```python
from build123d import *

# Parameters (mm, degrees)
BOSS_EXTRU_1_DEPTH = 10


with BuildPart() as part:
    # Esquisse1 → Boss.-Extru.1 (new body)
    with BuildSketch(Plane(origin=(0, 0, 0), x_dir=(1, 0, 0), z_dir=(0, 1, 0))):
        with BuildLine():
            Line((112.426746773, 8.058530984), (208.426746773, 8.058530984))
            Line((208.426746773, 8.058530984), (214.268189678, 17.812491045))
            ThreePointArc((214.268189678, 17.812491045), (206.831645665, 27.458673867), (208.340233589, 39.544830921))
            Line((208.340233589, 39.544830921), (290.262052013, 184.417099293))
            ThreePointArc((290.262052013, 184.417099293), (299.910234809, 191.958577714), (312.065160821, 190.468912764))
            Line((312.065160821, 190.468912764), (318.76181291, 202.523064381))
            Line((318.76181291, 202.523064381), (269.51839591, 284.931109389))
            Line((269.51839591, 284.931109389), (258.259283583, 284.517680144))
            Line((258.259283583, 284.517680144), (258.259283583, 282.707559459))
            ThreePointArc((258.259283583, 282.707559459), (253.572992082, 271.39385096), (242.259283583, 266.707559459))
            Line((242.259283583, 266.707559459), (75.828641942, 266.707559459))
            ThreePointArc((75.828641942, 266.707559459), (64.656934191, 271.253610536), (59.833620697, 282.308441218))
            Line((59.833620697, 282.308441218), (59.827222367, 282.56486004))
            Line((59.827222367, 282.56486004), (48.463462476, 282.281304065))
            Line((48.463462476, 282.281304065), (1.209576466, 198.716537226))
            Line((1.209576466, 198.716537226), (7.119810651, 189.400838648))
            ThreePointArc((7.119810651, 189.400838648), (19.083596298, 190.931024082), (28.716557185, 183.672945892))
            Line((28.716557185, 183.672945892), (114.087531018, 40.806031234))
            ThreePointArc((114.087531018, 40.806031234), (115.621763688, 27.817531222), (106.953563168, 18.023793314))
            Line((106.953563168, 18.023793314), (112.426746773, 8.058530984))
        make_face()
    extrude(amount=BOSS_EXTRU_1_DEPTH)


solid = part.part
```
Input: part model. Units: mm. Frame: model coordinates. A direction names the side the tool comes from. Round coordinates to 2 decimals unless told otherwise and drop trailing zeros. Write each loop counter-clockwise with the first axis right and the second up, starting at its lowest first coordinate (ties: lowest second). Pieces come first, ordered by that corner, then holes. Notation, with made-up numbers: M 33.5,53.5 L 85.5,53.5 A23 cw 85.5,65.5 Z; hole C 75,41 d2. An arc over 180 degrees is marked long. Write each question's results on one line, items separated by ' | '.
Q1. Draft query along X for faces 3 (the face through (160, 5, -266.708)), 4 (the face through (294.485, 4.93, -243.15)), 5 (the face through (158, 0, -148)). Return one class per face: released by +X, released by -X, zero draft, split by the parting line, or undercut.
Results:
face 3: undercut | face 4: released by +X | face 5: zero draft
Q2. Line query: line 1 along Z through (x, y) = (179, 1.25); line 2 along Z through (x, y) = (84, 3.5); line 3 along X through (y, z) = (9.75, -82.5). Output: solid intervals per line, ascending.
Results:
line 1: z = -266.71 to -8.06 | line 2: z = -266.71 to -91.16 | line 3: x = 89.17 to 232.63
Q3. Access query for faces 1 (the face through (263.968, 4.93, -284.727)), 2 (the face through (253.7, 4.93, -271.52)). Directions: +Z, -Z, +X, -X, +Y, -Y. A direction counts if a zero-diameter tool reaches every point of the face in a straight line with its end or side. Return the directions, or none.
Results:
face 1: -Z, -X, +Y, -Y | face 2: -Z, +Y, -Y
Q4. Pin query (flat end, axial travel): P1, Ø3, axis at x = 283, y = 7, coming from the +Z side; P2, Ø1.5, axis at x = 105, y = 6.5, coming from the +Z side; P3, Ø0.5, axis at y = 5.5, z = -284, coming from the -X side. Return the tip coordinate at first contact, or that it passes through.
Results:
P1: stops at z = -168.92 | P2: stops at z = -54.76 | P3: stops at x = 258.26
Q5. Section query B-B (x = 181). Return loops of the section in (y, z), and give its area (3 significant figures).
Results:
outline: M 0,-266.71 L 10,-266.71 L 10,-8.06 L 0,-8.06 Z | area: 2,590 mm^2
Q6. Section query C-C (z = -262). Return loops of the section in (x, y).
Results:
outline: M 36.99,0 L 283.22,0 L 283.22,10 L 36.99,10 Z
Q7. Section query A-A (y = 7.5). Return loops of the section in (x, z).
Results:
outline: M 1.21,-198.72 L 48.46,-282.28 L 59.83,-282.56 L 59.83,-282.31 A16 cw 75.83,-266.71 L 242.26,-266.71 A16 cw 258.26,-282.71 L 258.26,-284.52 L 269.52,-284.93 L 318.76,-202.52 L 312.07,-190.47 A16 cw 290.26,-184.42 L 208.34,-39.54 A16 cw 214.27,-17.81 L 208.43,-8.06 L 112.43,-8.06 L 106.95,-18.02 A16 cw 114.09,-40.81 L 28.72,-183.67 A16 cw 7.12,-189.4 Z
